```python
from build123d import *

# Parameters (mm, degrees)
EXTRUDE_1_DEPTH    = 4
SKETCH_2_R         = 5
EXTRUDE_2_DEPTH    = 1.9
HOLE_WIZARD_M6_1_D = 5
FILLET_1_R         = 0.5


with BuildPart() as part:
    # 草图1 → 凸台-拉伸1 (new body)
    with BuildSketch(Plane.XY):
        Polygon((5.773502692, 0), (2.886751346, 5), (-2.886751346, 5), (-5.773502692, 0), (-2.886751346, -5), (2.886751346, -5), align=None)
    extrude(amount=EXTRUDE_1_DEPTH)

    # 草图2 → 凸台-拉伸2 (add)
    with BuildSketch(Plane.XY.offset(4)):
        with Locations(Location((0, 0, 0), (0, 0, 210))):
            Circle(SKETCH_2_R)
    extrude(amount=EXTRUDE_2_DEPTH)

    # M6 螺纹孔1 (through all)
    with Locations(Plane.XY.offset(5.9)):
        with Locations((0, 0)):
            Hole(HOLE_WIZARD_M6_1_D / 2)

    # 圆角1
    fillet_1_edges = [part.edges().sort_by_distance(p)[0] for p in [
        (4.330127019, 2.5, 5.9),
    ]]
    fillet(fillet_1_edges, radius=FILLET_1_R)


solid = part.part
```
Geometry: final body of the model. Coordinates: model frame, mm. A direction names the side the tool comes from. Round coordinates to 2 decimals unless told otherwise and drop trailing zeros. Loops run counter-clockwise (first coordinate to the right, second up) from the corner with the lowest first, then second, coordinate; pieces in that order, holes last.
Item 1: Line query: L1, parallel to Y at x = 0, z = 3.5; L2, parallel to X at y = -1.75, z = 2.4; L3, parallel to X at y = -1, z = 3. Output: solid intervals per line, ascending.
Checked values:
L1: y = -5 to -2.5, 2.5 to 5
L2: x = -4.76 to -1.79, 1.79 to 4.76
L3: x = -5.2 to -2.29, 2.29 to 5.2
Item 2: Mould query, pull axis X, two halves, no side actions, for faces 5 (the cylindrical face through (3, -4, 5)), 6 (the cylindrical face through (0.54, -2.44, 2.91)), 7 (the flat face through (4.35, 2.465, 1.972)). Classes: released by +X, released by -X, zero draft, split by the parting line, or undercut.
Checked values:
face 5: split by the parting line
face 6: undercut
face 7: released by +X
Item 3: Contact query for flat-ended pins moving along their axis: P1, Ø1, axis at y = 2.5, z = 2.5, coming from the +X side; P2, Ø0.7, axis at x = -2.5, y = 4.5, coming from the +Z side. Output: stop coordinate, or through.
Checked values:
P1: stops at x = 4.62
P2: stops at z = 5.8
Item 4: Section B-B, the plane z = 4.25. Output: boundary loops of the cut face in (x, y).
Checked values:
outline: circle Ø10 at (0, 0); hole circle Ø5 at (0, 0)
Item 5: Reachability of faces 1 (the flat face through (-2.7, 4.5, 4)), 2 (the flat face through (2.6, -4.5, 4)), 3 (the flat face through (-2.7, -4.5, 4)), 4 (the flat face through (2.6, 4.5, 4)) from +Z, -Z, +X, -X, +Y, -Y: full face, straight path, thin tool, end or side. Return the list, or none.
Checked values:
face 1: +Z, -X, +Y
face 2: +Z, +X, -Y
face 3: +Z, -X, -Y
face 4: +Z, +X, +Y
Item 6: Section A-A, the plane z = 1.9. Output: boundary loops of the cut face in (x, y).
Checked values:
outline: (-5.77, 0) - (-2.89, -5) - (2.89, -5) - (5.77, 0) - (2.89, 5) - (-2.89, 5) - close; hole circle Ø5 at (0, 0)
